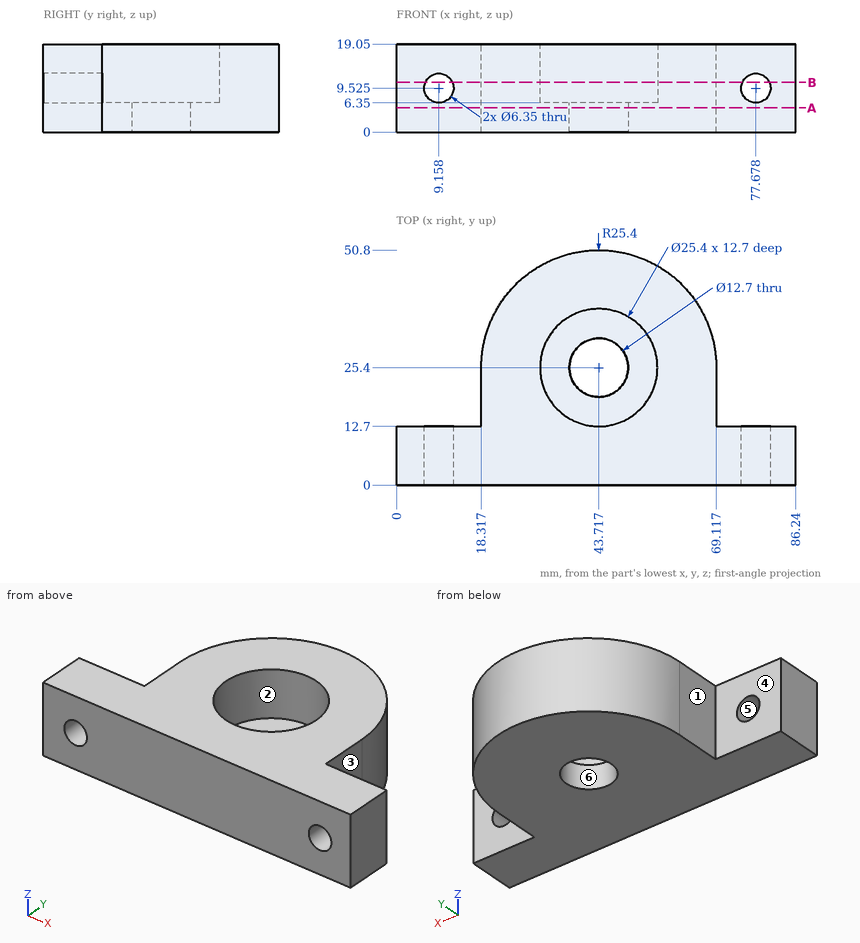
Study the drawing (mm; zero at the part's minimum x, y, z) and answer. A direction names the side the tool comes from. Give positions to 0.01 mm unless a question says otherwise; leave off trailing zeros. Write each loop counter-clockwise with the first axis right and the second up, starting at its lowest first coordinate (ties: lowest second). Pieces come first, ordered by that corner, then holes. Notation, with made-up numbers: (40, 43) - (94, 43) arc R18 ccw to (94, 74) - close; hole circle Ø5 at (4, 20.25). An arc over 180 degrees is marked (long way). One line per question, with ' | ' between items. Start each with the question number.
1. For the marked faces 1, 2 and 3, determine the directions among +Z, -Z, +X, -X, +Y, -Y from which every point of the face is accessible in a straight line to the end or side of a thin tool.
2. Determine the mould class of the marked faces 4, 5 and 6 for opening direction Y: +Y half, -Y half, draft (parallel to the pull), parting line (faces both ways), or undercut.
3. Section B-B, the plane z = 10.75 is taken. Determine the outline of the cut face in (x, y).
4. Section A-A, the plane z = 5.25 is taken. Determine the outline of the cut face in (x, y).
5. Straight lines are drawn through the part: line 1 (X direction, y = 3, z = 9.5); line 2 (X direction, y = 9, z = 8.75); line 3 (Y direction, x = 44, z = 4.25). For each, find the intervals that lie inside material, in ascending order.
6. Given P1, Ø8.5, axis at x = 79.5, z = 7, coming from the +Y side; P2, Ø1.5, axis at x = 45, y = 35.5, coming from the +Z side; P3, Ø3, axis at x = 33, z = 3.5, coming from the +Y side, each flat-ended and moving along its own axis, determine where each tip first touches the part or whether it passes through.
Result:
1) face 1: +Z, -Z, -X, +Y | face 2: +Z | face 3: +Z, -Z, +X, +Y
2) face 4: +Y half | face 5: draft | face 6: undercut
3) outline: (0, 0) - (6.23, 0) - (6.23, 12.7) - (0, 12.7) - close; (12.09, 0) - (74.75, 0) - (74.75, 12.7) - (69.12, 12.7) - (69.12, 25.4) arc R25.4 ccw to (18.32, 25.4) - (18.32, 12.7) - (12.09, 12.7) - close; (80.61, 0) - (86.24, 0) - (86.24, 12.7) - (80.61, 12.7) - close; hole circle Ø25.4 at (43.72, 25.4)
4) outline: (0, 0) - (86.24, 0) - (86.24, 12.7) - (69.12, 12.7) - (69.12, 25.4) arc R25.4 ccw to (18.32, 25.4) - (18.32, 12.7) - (0, 12.7) - close; hole circle Ø12.7 at (43.72, 25.4)
5) line 1: x = 0 to 5.98, 12.33 to 74.5, 80.85 to 86.24 | line 2: x = 0 to 6.08, 12.24 to 74.6, 80.76 to 86.24 | line 3: y = 0 to 19.06, 31.74 to 50.8
6) P1: stops at y = 12.7 | P2: stops at z = 6.35 | P3: stops at y = 49.07
